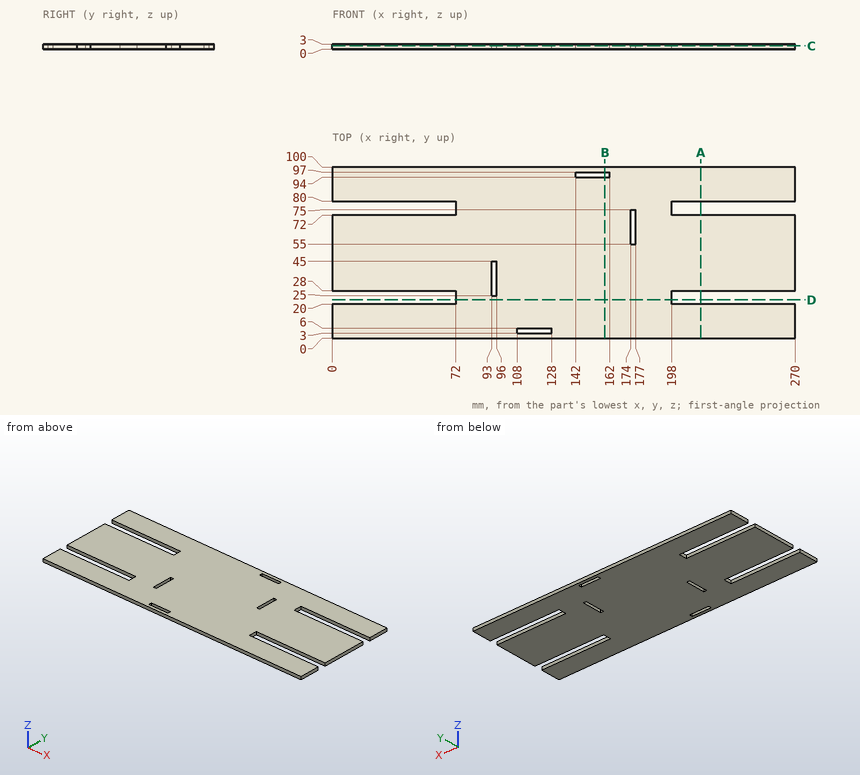
Verification items for this drawing (mm, ordinates from the low corner). Coordinates: 2 decimals unless noted, no trailing zeros. Loops run counter-clockwise (first coordinate to the right, second up) from the corner with the lowest first, then second, coordinate; pieces in that order, holes last.
Item 1: Sectioned sample at C-C, the plane z = 1.85. Count the separate pieces of the cut face and the enclosed holes in it, then the cut area to 3 significant figures.
Item 2: Thickness scan on line 1 (Y direction, x = 14.5, z = 0.55); line 2 (X direction, y = 40.5, z = 0.65); line 3 (Y direction, x = 157, z = 1.6). Record the ranges inside material, lowest first.
Item 3: Sectioned sample at B-B, the plane x = 159. Record the boundary of the cut face in (y, z).
Item 4: Go/stop test with flat-tipped pins: pin 1 Ø1.5 at (y, z) = (22, 2) entering from -X; pin 2 Ø0.9 at (y, z) = (22, 2) entering from +X. Record where each tip stops, or that it passes through.
Item 5: Sectioned sample at A-A, the plane x = 215. Record the boundary of the cut face in (y, z), then the cut area to 3 significant figures.
Item 6: Sectioned sample at D-D, the plane y = 22.5. Record the boundary of the cut face in (x, z), then the cut area to 3 significant figures.
Check result:
1. separate pieces: 1
1. enclosed holes: 4
1. area: 24,500 mm2
2. line 1: y = 0 to 20, 28 to 72, 80 to 100
2. line 2: x = 0 to 93, 96 to 270
2. line 3: y = 0 to 94, 97 to 100
3. outline: (0, 0) - (94, 0) - (94, 3) - (0, 3) - close; (97, 0) - (100, 0) - (100, 3) - (97, 3) - close
4. pin 1: stops at x = 72
4. pin 2: stops at x = 198
5. outline: (0, 0) - (20, 0) - (20, 3) - (0, 3) - close; (28, 0) - (72, 0) - (72, 3) - (28, 3) - close; (80, 0) - (100, 0) - (100, 3) - (80, 3) - close
5. area: 252 mm2
6. outline: (72, 0) - (198, 0) - (198, 3) - (72, 3) - close
6. area: 378 mm2
